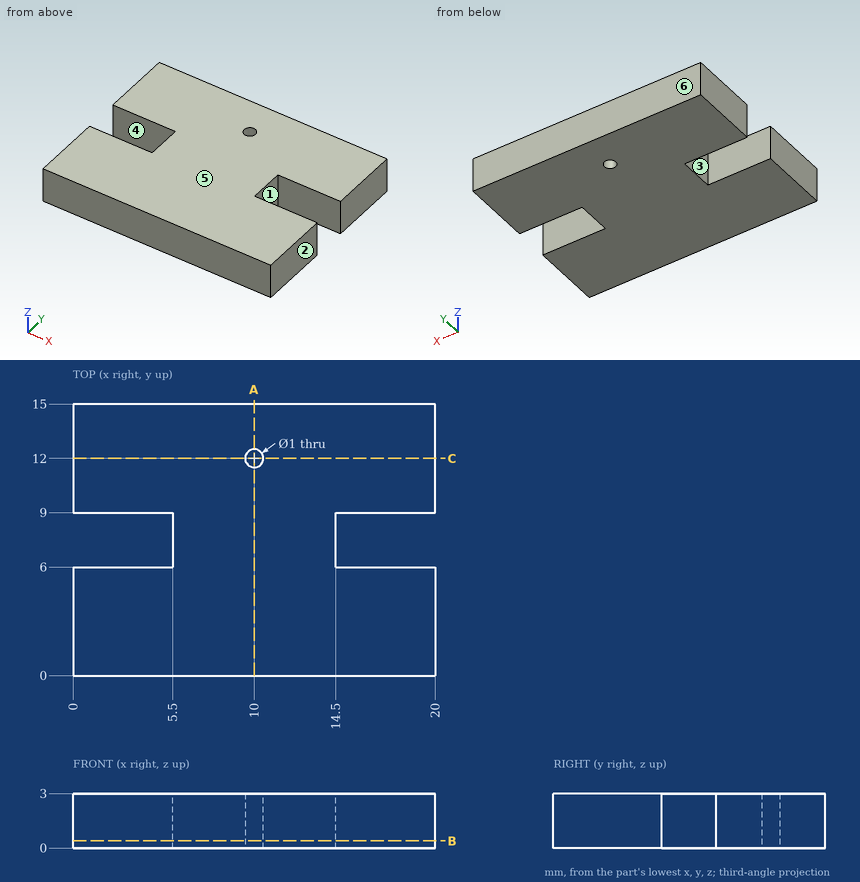
For this review, use the dimensioned drawing (mm, ordinates from the lowest corner) and the shaded views. A direction names the side the tool comes from. Round coordinates to 2 decimals unless told otherwise and drop trailing zeros. Write each loop counter-clockwise with the first axis right and the second up, starting at its lowest first coordinate (ties: lowest second). Pieces come first, ordered by that corner, then holes. Notation, with made-up numbers: (56.25, -1) - (114.25, -1) arc R24 cw to (114.25, 37) - close; hole circle Ø9 at (-11.5, -1). An arc over 180 degrees is marked (long way). Use a Markdown table: item, result.
Q1. The part is to be moulded in two halves that separate along Y. For the marked faces 4, 5 and 6, say which applies: pulls with the +Y half, pulls with the -Y half, needs draft (parallel to the pull), parting line crosses it, or undercut.
Derived:
| item | result |
|---|---|
| face 4 | undercut |
| face 5 | needs draft |
| face 6 | pulls with the +Y half |
Q2. Machinability: for the marked faces 1, 2 and 3, which of the approach directions +Z, -Z, +X, -X, +Y, -Y give a long, thin tool a straight path to every point of the face, cutting with its end or side? Answer none if there is none.
Derived:
| item | result |
|---|---|
| face 1 | +Z, -Z, +X |
| face 2 | +Z, -Z, +X, +Y, -Y |
| face 3 | +Z, -Z, -X |
Q3. Clearance check with flat-ended pins moving along their axes: pin 1 (0.9 mm diameter, centred on y = 7.5, z = 1.5, fed in from +X); pin 2 (0.9 mm diameter, centred on y = 8, z = 1, fed in from -X). State where each tip first meets the part, or that it passes through.
Derived:
| item | result |
|---|---|
| pin 1 | stops at x = 14.5 |
| pin 2 | stops at x = 5.5 |
Q4. We need section C-C (y = 12). Give the boundary of the cut face in (x, z).
Derived:
| item | result |
|---|---|
| outline | (0, 0) - (9.5, 0) - (9.5, 3) - (0, 3) - close; (10.5, 0) - (20, 0) - (20, 3) - (10.5, 3) - close |
Q5. Wall thickness on line 1 along Y through (x, z) = (10, 1.55); line 2 along Y through (x, z) = (16, 0.3); line 3 along X through (y, z) = (6.75, 1.05): over which ranges is each line inside the solid? List them lowest first.
Derived:
| item | result |
|---|---|
| line 1 | y = 0 to 11.5, 12.5 to 15 |
| line 2 | y = 0 to 6, 9 to 15 |
| line 3 | x = 5.5 to 14.5 |
Q6. We need section B-B (z = 0.4). Give the boundary of the cut face in (x, y).
Derived:
| item | result |
|---|---|
| outline | (0, 0) - (20, 0) - (20, 6) - (14.5, 6) - (14.5, 9) - (20, 9) - (20, 15) - (0, 15) - (0, 9) - (5.5, 9) - (5.5, 6) - (0, 6) - close; hole circle Ø1 at (10, 12) |
Q7. We need section A-A (x = 10). Give the boundary of the cut face in (y, z).
Derived:
| item | result |
|---|---|
| outline | (0, 0) - (11.5, 0) - (11.5, 3) - (0, 3) - close; (12.5, 0) - (15, 0) - (15, 3) - (12.5, 3) - close |
